The listing builds one solid part. Answer for the finished solid, in the listing's coordinates (mm). A direction names the side the tool comes from. Coordinates: 2 decimals unless noted, no trailing zeros. Order: outer loops, then holes, each group sorted by start corner. A loop starts at its lowest first (then second) coordinate and runs counter-clockwise, first axis right, second up. Notation, with made-up numbers: (84, 81) -> (115, 81) arc R22 cw to (115, 87) -> close; hole circle Ø10 at (58.5, 65.5). An arc over 180 degrees is marked (long way). One line per question, with ' | ' between items.
from build123d import *

# Parameters (mm, degrees)
SPROCKET_R                   = 45
ESTRUSIONE_ESTRUSIONE2_DEPTH = 8
TAGLIO_ESTRUSIONE1_DEPTH     = 9
RACCORDO1_R                  = 3.5
SCHIZZO1_R                   = 5
SCHIZZO1_R_2                 = 1.5
TAGLIO_ESTRUSIONE2_DEPTH     = 9
TAGLIO_ESTRUSIONE3_DEPTH     = 9


with BuildPart() as part:
    # Sprocket → Estrusione-Estrusione2 (new body)
    with BuildSketch(Plane(origin=(0, 0, 0), x_dir=(0, 0, -1), z_dir=(1, 0, 0))):
        Circle(SPROCKET_R)
    extrude(amount=ESTRUSIONE_ESTRUSIONE2_DEPTH)

    # Tooth → Taglio-Estrusione1 (cut, through all)
    with BuildSketch(Plane(origin=(0, 0, 0), x_dir=(0, 0, -1), z_dir=(1, 0, 0))):
        Polygon((-5, 45), (5, 45), (1.75, 36), (-1.75, 36), align=None)
        Polygon((24.0296126, 38.37418036), (17.196510127, 31.675582701), (14.043119089, 33.194175788), (15.019923921, 42.713017751), align=None)
        Polygon((38.29986572, 24.147883671), (29.237040522, 21.077427773), (27.054826216, 23.813837961), (32.064967702, 31.966198496), align=None)
        Polygon((44.984360718, 5.138802467), (35.486816473, 6.304629776), (34.707993204, 9.716877469), (42.759151378, 14.888081589), align=None)
        Polygon((42.759151378, -14.888081589), (34.707993204, -9.716877469), (35.486816473, -6.304629776), (44.984360718, -5.138802467), align=None)
        Polygon((32.064967702, -31.966198496), (27.054826216, -23.813837961), (29.237040522, -21.077427773), (38.29986572, -24.147883671), align=None)
        Polygon((15.019923921, -42.713017751), (14.043119089, -33.194175788), (17.196510127, -31.675582701), (24.0296126, -38.37418036), align=None)
        Polygon((-5, -45), (-1.75, -36), (1.75, -36), (5, -45), align=None)
        Polygon((-24.0296126, -38.37418036), (-17.196510127, -31.675582701), (-14.043119089, -33.194175788), (-15.019923921, -42.713017751), align=None)
        Polygon((-38.29986572, -24.147883671), (-29.237040522, -21.077427773), (-27.054826216, -23.813837961), (-32.064967702, -31.966198496), align=None)
        Polygon((-44.984360718, -5.138802467), (-35.486816473, -6.304629776), (-34.707993204, -9.716877469), (-42.759151378, -14.888081589), align=None)
        Polygon((-42.759151378, 14.888081589), (-34.707993204, 9.716877469), (-35.486816473, 6.304629776), (-44.984360718, 5.138802467), align=None)
        Polygon((-32.064967702, 31.966198496), (-27.054826216, 23.813837961), (-29.237040522, 21.077427773), (-38.29986572, 24.147883671), align=None)
        Polygon((-15.019923921, 42.713017751), (-14.043119089, 33.194175788), (-17.196510127, 31.675582701), (-24.0296126, 38.37418036), align=None)
    extrude(amount=TAGLIO_ESTRUSIONE1_DEPTH, mode=Mode.SUBTRACT)

    # Raccordo1
    raccordo1_edges = [part.edges().sort_by_distance(p)[0] for p in [
        (4, -5.173509038, -44.701619705),
        (4, -14.734135321, -42.519469145),
        (4, -24.056476483, -38.030066253),
        (4, -31.723503477, -31.915816253),
        (4, 44.732070833, 4.903247801),
        (4, 44.732070833, -4.903247801),
        (4, -38.174763728, -23.826191772),
        (4, -42.429642707, -14.990844531),
        (4, -44.732070833, -4.903247801),
        (4, -44.732070833, 4.903247801),
        (4, -42.429642707, 14.990844531),
        (4, -38.174763728, 23.826191772),
        (4, -31.723503477, 31.915816253),
        (4, -24.056476483, 38.030066253),
        (4, -14.734135321, 42.519469145),
        (4, -5.173509038, 44.701619705),
        (4, 5.173509038, 44.701619705),
        (4, 14.734135321, 42.519469145),
        (4, 24.056476483, 38.030066253),
        (4, 31.723503477, 31.915816253),
        (4, 38.174763728, 23.826191772),
        (4, 42.429642707, 14.990844531),
        (4, 42.429642707, -14.990844531),
        (4, 38.174763728, -23.826191772),
        (4, 31.723503477, -31.915816253),
        (4, 24.056476483, -38.030066253),
        (4, 14.734135321, -42.519469145),
        (4, 5.173509038, -44.701619705),
    ]]
    fillet(raccordo1_edges, radius=RACCORDO1_R)

    # Schizzo1 → Taglio-Estrusione2 (cut, through all)
    with BuildSketch(Plane(origin=(0, 0, 0), x_dir=(0, 0, -1), z_dir=(1, 0, 0))):
        Circle(SCHIZZO1_R)
        with Locations((0, 8)):
            Circle(SCHIZZO1_R_2)
        with Locations((8, 0)):
            Circle(SCHIZZO1_R_2)
        with Locations((0, -8)):
            Circle(SCHIZZO1_R_2)
        with Locations((-8, 0)):
            Circle(SCHIZZO1_R_2)
        with Locations((0, 23)):
            Circle(SCHIZZO1_R_2)
        with Locations((23, 0)):
            Circle(SCHIZZO1_R_2)
        with Locations((0, -23)):
            Circle(SCHIZZO1_R_2)
        with Locations((-23, 0)):
            Circle(SCHIZZO1_R_2)
    extrude(amount=TAGLIO_ESTRUSIONE2_DEPTH, mode=Mode.SUBTRACT)

    # Schizzo2 → Taglio-Estrusione3 (cut, through all)
    with BuildSketch(Plane(origin=(8, 0, 0), x_dir=(0, 0, -1), z_dir=(1, 0, 0))):
        with BuildLine():
            Line((-26.83281573, 8), (-8, 8))
            Line((-8, 8), (-8, 26.83281573))
            ThreePointArc((-8, 26.83281573), (-19.798989873, 19.798989873), (-26.83281573, 8))
        make_face()
        with BuildLine():
            Line((26.83281573, 8), (8, 8))
            Line((8, 8), (8, 26.83281573))
            ThreePointArc((8, 26.83281573), (19.798989873, 19.798989873), (26.83281573, 8))
        make_face()
        with BuildLine():
            Line((8, -26.83281573), (8, -8))
            Line((8, -8), (26.83281573, -8))
            ThreePointArc((26.83281573, -8), (19.798989873, -19.798989873), (8, -26.83281573))
        make_face()
        with BuildLine():
            Line((-26.83281573, -8), (-8, -8))
            Line((-8, -8), (-8, -26.83281573))
            ThreePointArc((-8, -26.83281573), (-19.798989873, -19.798989873), (-26.83281573, -8))
        make_face()
    extrude(amount=-TAGLIO_ESTRUSIONE3_DEPTH, mode=Mode.SUBTRACT)


solid = part.part
Item 1: Each of these flat-tipped pins is pushed along its axis until it touches: pin 1 Ø4 at (x, y) = (2, 17) entering from -Z; pin 2 Ø2.5 at (y, z) = (0, 23) entering from -X; pin 3 Ø4 at (x, z) = (2.5, -17) entering from -Y; pin 4 Ø2.5 at (x, z) = (5, -16) entering from +Y. Where does it stop, or does it pass through?
Computed values:
pin 1: stops at z = -41.73 | pin 2: passes through | pin 3: stops at y = -33.44 | pin 4: stops at y = 32.85
Item 2: Determine the mould class of faces 4 (the face through (3.944, -21.513, 0.195)), 5 (the face through (3.944, 37.175, -24.013)), 6 (the face through (3.94, -19.55, -40.53)), 7 (the face through (4, 8, 18)) for opening direction Y: pulls with the +Y half, pulls with the -Y half, needs draft (parallel to the pull), parting line crosses it, or undercut.
Computed values:
face 4: undercut | face 5: pulls with the +Y half | face 6: pulls with the -Y half | face 7: undercut
Item 3: Section B-B, the plane z = 0 is taken. Give the vertices of the cut face in (x, y), plus the area to 3 significant figures.
Computed values:
outline: (0, -36) -> (8, -36) -> (8, -24.5) -> (0, -24.5) -> close; (0, -21.5) -> (8, -21.5) -> (8, -9.5) -> (0, -9.5) -> close; (0, -6.5) -> (8, -6.5) -> (8, -5) -> (0, -5) -> close; (0, 5) -> (8, 5) -> (8, 6.5) -> (0, 6.5) -> close; (0, 9.5) -> (8, 9.5) -> (8, 21.5) -> (0, 21.5) -> close; (0, 24.5) -> (8, 24.5) -> (8, 36) -> (0, 36) -> close | area: 400 mm^2
Item 4: For faces 1 (the face through (3.94, -43.88, -9.98)), 2 (the face through (4, -17, 8)), 3 (the face through (3.944, 5.907, -38.726)), determine the directions among +Z, -Z, +X, -X, +Y, -Y from which every point of the face is accessible in a straight line to the end or side of a thin tool.
Computed values:
face 1: -Z, +X, -X, -Y | face 2: +X, -X | face 3: -Z, +X, -X
Item 5: Section C-C, the plane z = -38.5 is taken. Give the vertices of the cut face in (x, y).
Computed values:
outline: (0, -22.67) -> (8, -22.67) -> (8, -12.15) -> (0, -12.15) -> close; (0, -5.93) -> (8, -5.93) -> (8, 5.93) -> (0, 5.93) -> close; (0, 12.15) -> (8, 12.15) -> (8, 22.67) -> (0, 22.67) -> close
Item 6: Section A-A, the plane y = 0 is taken. Give the vertices of the cut face in (x, z).
Computed values:
outline: (0, -45) -> (8, -45) -> (8, -24.5) -> (0, -24.5) -> close; (0, -21.5) -> (8, -21.5) -> (8, -9.5) -> (0, -9.5) -> close; (0, -6.5) -> (8, -6.5) -> (8, -5) -> (0, -5) -> close; (0, 5) -> (8, 5) -> (8, 6.5) -> (0, 6.5) -> close; (0, 9.5) -> (8, 9.5) -> (8, 21.5) -> (0, 21.5) -> close; (0, 24.5) -> (8, 24.5) -> (8, 45) -> (0, 45) -> close
Item 7: Section D-D, the plane x = 5.75 is taken. Count the separate pieces of the cut face and the enclosed holes in it, plus the area to 3 significant figures.
Computed values:
separate pieces: 1 | enclosed holes: 13 | area: 4,390 mm^2
Item 8: Find the intervals of material crossed by L1, parallel to Z at x = 4.25, y = 21; L2, parallel to Y at x = 4, z = 0; L3, parallel to Z at x = 7.25, y = 1, in increasing order.
Computed values:
L1: z = -39.8 to -18.52, -8 to 8, 18.52 to 39.8 | L2: y = -36 to -24.5, -21.5 to -9.5, -6.5 to -5, 5 to 6.5, 9.5 to 21.5, 24.5 to 36 | L3: z = -44.99 to -24.12, -21.88 to -9.12, -6.88 to -4.9, 4.9 to 6.88, 9.12 to 21.88, 24.12 to 44.99
